Can you work these out from the model? Positions are in its coordinate system, mm. Face numbers are marked on the shaded views. Coordinates: 2 decimals unless noted, no trailing zeros. Write each loop counter-clockwise with the first axis right and the second up, starting at its lowest first coordinate (ties: lowest second). Pieces come first, ordered by that corner, then holes.
```python
from build123d import *

# Parameters (mm, degrees)
CUT_EXTRUDE1_START = -9.525
CUT_EXTRUDE1_DEPTH = 9.525
CIRPATTERN1_COUNT  = 12


with BuildPart() as part:
    # Sketch2 → Revolve1 (revolve)
    with BuildSketch(Plane.XY, mode=Mode.PRIVATE) as revolve1_sk:
        Polygon((-22.225, 57.15), (-9.525, 57.15), (-9.525, 52.3875), (-1.7653, 52.3875), (-1.7653, 49.022), (1.7653, 49.022), (1.7653, 52.3875), (9.525, 52.3875), (9.525, 34.925), (-22.225, 34.925), align=None)
    revolve(revolve1_sk.sketch.rotate(Axis((0, 0, 0), (1, 0, 0)), 90), axis=Axis((0, 0, 0), (1, 0, 0)))

    # Sketch3 → Cut-Extrude1 (cut)
    with BuildSketch(Plane.ZY.offset(22.225).offset(CUT_EXTRUDE1_START)):
        with BuildLine():
            Line((-4.7625, 56.951216789), (-4.7625, 50.576265123))
            ThreePointArc((-4.7625, 50.576265123), (0, 50.8), (4.7625, 50.576265123))
            Line((4.7625, 50.576265123), (4.7625, 56.951216789))
            ThreePointArc((4.7625, 56.951216789), (0, 57.15), (-4.7625, 56.951216789))
        make_face()
    cut_extrude1 = extrude(amount=CUT_EXTRUDE1_DEPTH, mode=Mode.SUBTRACT)

    # CirPattern1: Cut-Extrude1 ×12 about axis
    cirpattern1_axis = Axis((0, 0, 0), (1, 0, 0))
    for i in range(1, CIRPATTERN1_COUNT):
        add(cut_extrude1.rotate(cirpattern1_axis, i * 360 / CIRPATTERN1_COUNT), mode=Mode.SUBTRACT)


solid = part.part
```
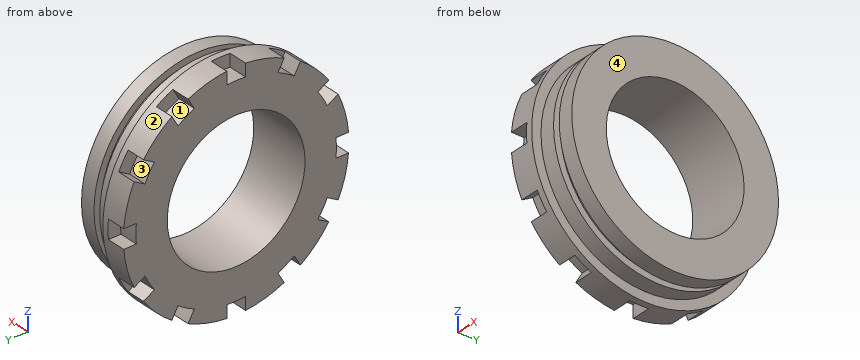
1. We'd pull the mould along Y, two halves only. Please class the marked faces 1, 2, 3 and 4: released by +Y, released by -Y, zero draft, split by the parting line, or undercut.
2. If we section it at A-A, the plane z = 14.5: List the corners of the cut face in (x, y) for me (3 decimals), plus the area to 3 significant figures.
3. If I drill on L1, parallel to Y at x = -14, z = 0 (3 decimals); L2, parallel to Y at x = -2.5, z = 0 (1 decimal); L3, parallel to X at y = -29, z = -49 (3 decimals), over which ranges is the centre line in solid material (lowest first)?
4. I'm going to push flat-ended pins straight in: P1, Ø3, axis at x = -5, y = -14, coming from the -Z side; P2, Ø4, axis at x = 1.5, y = -34, coming from the -Z side; P3, Ø3, axis at x = -19.5, z = 53, coming from the +Y side. Where does each tip first touch, or does it pass through?
Answers:
1. face 1: undercut
1. face 2: split by the parting line
1. face 3: undercut
1. face 4: zero draft
2. outline: (-22.225, -55.28) - (-9.525, -55.28) - (-9.525, -50.341) - (-1.765, -50.341) - (-1.765, -46.828) - (1.765, -46.828) - (1.765, -50.341) - (9.525, -50.341) - (9.525, -31.773) - (-22.225, -31.773) - close; (-22.225, 31.773) - (9.525, 31.773) - (9.525, 50.341) - (1.765, 50.341) - (1.765, 46.828) - (-1.765, 46.828) - (-1.765, 50.341) - (-9.525, 50.341) - (-9.525, 55.28) - (-22.225, 55.28) - close
2. area: 1,280 mm2
3. L1: y = -50.8 to -34.925, 34.925 to 50.8
3. L2: y = -52.4 to -34.9, 34.9 to 52.4
3. L3: x = -12.7 to -9.525
4. P1: stops at z = -50.87
4. P2: stops at z = -41.46
4. P3: stops at y = 24.35
